Part model, mm, in its own coordinate system. A direction names the side the tool comes from. Round coordinates to 2 decimals unless told otherwise and drop trailing zeros. Write each loop counter-clockwise with the first axis right and the second up, starting at its lowest first coordinate (ties: lowest second). Pieces come first, ordered by that corner, then holes. Notation, with made-up numbers: M 18,75 L 74,75 A21 cw 74,96 Z; hole C 87.25,14 d10. An arc over 180 degrees is marked long. Use one line per item in the form item = value. Start each with the question number.
Item 1: Flat gauge pins, fed straight in: pin 1 Ø0.8 at (y, z) = (-1, 17.5) entering from -X; pin 2 Ø0.5 at (x, y) = (15, -1) entering from +Z; pin 3 Ø0.5 at (y, z) = (-1, 20) entering from +X. Where does each tip first touch, or does it go through?
Item 2: Cut at D-D, the plane x = 27.5. Give the cut face in (y, z), then the cut area to 3 significant figures.
Item 3: Cut at C-C, the plane x = 15. Give the cut face in (y, z), then the cut area to 3 significant figures.
Item 4: Which spindle directions (+Z, -Z, +X, -X, +Y, -Y) get a long thin tool onto all of the face, cutting with end or side? Do faces 4 (the face through (24.801, 0.715, 15.394)), 5 (the face through (11.7, -1.5, -0.3)), 6 (the face through (1.5, -1, 15)), 7 (the face through (24.785, -2.199, 15.106)). Say none if no direction does.
Item 5: Cut at A-A, the plane z = 18.5. Give the cut face in (x, y), then the cut area to 3 significant figures.
Item 6: Cut at B-B, the plane y = -0.95. Give the cut face in (x, z).
Item 7: Mould opens along Y. For faces 1 (the face through (26, -1, 15)), 2 (the face through (13, -2.5, 0)), 3 (the face through (-0.719, -1.993, -0.594)) say: +Y half, -Y half, draft (parallel to the pull), parting line (faces both ways), or undercut.
Item 8: Probe L1, parallel to X at y = -1.05, z = 23.5; L2, parallel to Z at x = 19.5, y = 0.1; L3, parallel to X at y = -2.1, z = 19. List the from-to ranges inside material, lowest first.
from build123d import *

# Parameters (mm, degrees)
F1_DEPTH = 1.5
F3_DEPTH = 1
F5_DEPTH = 1
F6_R     = 0.99999


# Not quite as in the source:
# - a fillet or chamfer is up to 0.001 mm smaller than in the source, because OpenCascade refuses the exact size
# - ends of sketch curves that miss each other by under 0.0002 mm in the source are joined


with BuildPart() as f1:
    # F0 (on Front) → F1 (new body)
    with BuildSketch(Plane.XZ):
        with BuildLine():
            Line((1.5, 25.5), (0, 25.5))
            Line((0, 25.5), (0, 5))
            ThreePointArc((0, 5), (1.4644660941, 1.4644660941), (5, 0))
            Line((5, 0), (21, 0))
            ThreePointArc((21, 0), (24.5355339059, 1.4644660941), (26, 5))
            Line((26, 5), (26, 25.5))
            Line((26, 25.5), (24.5, 25.5))
            Line((24.5, 25.5), (24.5, 5))
            ThreePointArc((24.5, 5), (23.4748737342, 2.5251262658), (21, 1.5))
            Line((21, 1.5), (5, 1.5))
            ThreePointArc((5, 1.5), (2.5251262658, 2.5251262658), (1.5, 5))
            Line((1.5, 5), (1.5, 25.5))
        make_face()
    extrude(amount=F1_DEPTH)

    # F2 (on face) → F3 (join)
    with BuildSketch(Plane.XZ.offset(1.5)):
        with BuildLine():
            Line((1.5, 5), (1.5, 25.5))
            Line((1.5, 25.5), (-3, 25.5))
            Line((-3, 25.5), (-3, 4.9999991806))
            ThreePointArc((-3, 4.9999991806), (-0.6568544895, -0.6568544895), (4.9999991806, -3))
            Line((4.9999991806, -3), (21, -3))
            ThreePointArc((21, -3), (26.6568542495, -0.6568542495), (29, 5))
            Line((29, 5), (29, 25.5))
            Line((29, 25.5), (24.5, 25.5))
            Line((24.5, 25.5), (24.5, 5))
            ThreePointArc((24.5, 5), (23.4748737342, 2.5251262658), (21, 1.5))
            Line((21, 1.5), (5, 1.5))
            ThreePointArc((5, 1.5), (2.5251257362, 2.5251263156), (1.5, 5))
        make_face()
    extrude(amount=F3_DEPTH)

    # F4 (on face) → F5 (join)
    with BuildSketch(Plane(origin=(0, 0, 0), x_dir=(-1, 0, 0), z_dir=(0, 1, 0))):
        with BuildLine():
            Line((-24.5, 5), (-24.5, 25.5))
            Line((-24.5, 25.5), (-29, 25.5))
            Line((-29, 25.5), (-29, 5))
            ThreePointArc((-29, 5), (-26.6568542495, -0.6568542495), (-21, -3))
            Line((-21, -3), (-5, -3))
            ThreePointArc((-5, -3), (0.6568542495, -0.6568542495), (3, 5))
            Line((3, 5), (3, 25.5))
            Line((3, 25.5), (-1.5, 25.5))
            Line((-1.5, 25.5), (-1.5, 5))
            ThreePointArc((-1.5, 5), (-2.5251262658, 2.5251262658), (-5, 1.5))
            Line((-5, 1.5), (-21, 1.5))
            ThreePointArc((-21, 1.5), (-23.4748737342, 2.5251262658), (-24.5, 5))
        make_face()
    extrude(amount=F5_DEPTH)

    # F6 (radius 1 in the source; OpenCascade refuses exactly that, so slightly less here)
    f6_edges = [f1.edges().sort_by_distance(p)[0] for p in [
        (23.474874, 1, 2.525126),
        (24.5, -2.5, 15.25),
    ]]
    fillet(f6_edges, radius=F6_R)


solid = f1.part
Model answer:
q1.pin_1 = 0
q1.pin_2 = 1.5
q1.pin_3 = 26
q2.outline = M -2.5,0.34 L -1.5,0.34 L -1.5,25.5 L -2.5,25.5 Z; M 0,0.34 L 1,0.34 L 1,25.5 L 0,25.5 Z
q2.area = 50.3 mm²
q3.outline = M -2.5,-3 L -1.5,-3 L -1.5,0 L 0,0 L 0,-3 L 1,-3 L 1,0.5 A1 ccw 0,1.5 L -1.5,1.5 A1 ccw -2.5,0.5 Z
q3.area = 10.8 mm²
q4.face_4 = +Z, +Y
q4.face_5 = -Z
q4.face_6 = +Z, +Y, -Y
q4.face_7 = +Z, -Y
q5.outline = M -3,-2.5 L 0.5,-2.5 A1 ccw 1.5,-1.5 L 1.5,0 A1 ccw 0.5,1 L -3,1 L -3,0 L 0,0 L 0,-1.5 L -3,-1.5 Z; M 24.5,-1.5 A1 ccw 25.5,-2.5 L 29,-2.5 L 29,-1.5 L 26,-1.5 L 26,0 L 29,0 L 29,1 L 25.5,1 A1 ccw 24.5,0 Z
q5.area = 21.6 mm²
q6.outline = M 0,5 A5 ccw 5,0 L 21,0 A5 ccw 26,5 L 26,25.5 L 24.5,25.5 L 24.5,5 A3.5 cw 21,1.5 L 5,1.5 A3.5 cw 1.5,5 L 1.5,25.5 L 0,25.5 Z
q7.face_1 = undercut
q7.face_2 = -Y half
q7.face_3 = draft
q8.L1 = 0 to 1.5, 24.5 to 26
q8.L2 = -3 to 1.49
q8.L3 = -3 to 1.3, 24.7 to 29
